from build123d import *

# Parameters (mm, degrees)
F1_DEPTH = 6.35
F2_R     = 3.175
F3_DEPTH = 6.35
F5_DEPTH = 5


with BuildPart() as f1:
    # F0 (on Front) → F1 (new body)
    with BuildSketch(Plane.XZ):
        with BuildLine():
            Line((69.85, 12.7), (0, 12.7))
            ThreePointArc((0, 12.7), (-12.7, 0), (0, -12.7))
            Line((0, -12.7), (69.85, -12.7))
            ThreePointArc((69.85, -12.7), (82.55, 0), (69.85, 12.7))
        make_face()
    extrude(amount=F1_DEPTH)

    # F2 (on face) → F3 (cut, through all)
    with BuildSketch(Plane.XZ.offset(6.35)):
        Circle(F2_R)
        with Locations((24, 0)):
            Circle(F2_R)
    extrude(amount=-F3_DEPTH, mode=Mode.SUBTRACT)

    # F4 (on face) → F5 (cut)
    with BuildSketch(Plane(origin=(0, 0, 0), x_dir=(-1, 0, 0), z_dir=(0, 1, 0))):
        with BuildLine():
            Line((-23.55792, 7.161368), (-69.23386, 9.981001))
            ThreePointArc((-69.23386, 9.981001), (-79.85, 0), (-69.23386, -9.981001))
            Line((-69.23386, -9.981001), (-23.55792, -7.161368))
            ThreePointArc((-23.55792, -7.161368), (-16.825, 0), (-23.55792, 7.161368))
        make_face()
    extrude(amount=-F5_DEPTH, mode=Mode.SUBTRACT)


solid = f1.part
Could you check a few things on this model? Use its own coordinates, in mm. A direction names the side the tool comes from. Give positions to 0.01 mm unless a question says otherwise; leave off trailing zeros. Order: outer loops, then holes, each group sorted by start corner. A loop starts at its lowest first (then second) coordinate and runs counter-clockwise, first axis right, second up. Notation, with made-up numbers: (79.5, 1.5) -> (86.5, 1.5) arc R19 ccw to (86.5, 22.5) -> close; hole circle Ø6 at (84, 57). An arc over 180 degrees is marked (long way). Return JSON: item names as keys, results as strings.
1. Imagine slicing it at C-C on x = 63. List the corners of the cut face in (y, z) for me, then the cut area to 3 significant figures.
Answer list:
{"outline": "(-6.35, -12.7) -> (0, -12.7) -> (0, -9.6) -> (-5, -9.6) -> (-5, 9.6) -> (0, 9.6) -> (0, 12.7) -> (-6.35, 12.7) -> close", "area": "65.3 mm2"}
2. I need wall thicknesses on line 1 (Z direction, x = 0, y = -1.5) (3 decimals); line 2 (X direction, y = -0.5, z = -2.5); line 3 (Y direction, x = 34.5, z = 4.5). Which ranges of each line are inside material? Lowest first, please. Write a range as from..to.
Answer list:
{"line 1": "z = -12.7..-3.175, 3.175..12.7", "line 2": "x = -12.45..-1.96, 1.96..17.27, 79.53..82.3", "line 3": "y = -6.35..-5"}
3. For pin 1 Ø10 at (x, z) = (64.5, -2) entering from +Y, with a flat end and sliding along its axis, tell me the tip position at first contact or that it passes through.
Answer list:
{"pin 1": "stops at y = -5"}
4. Imagine slicing it at B-B on z = 0. List the corners of the cut face in (x, y) for me (3 decimals), then the cut area to 3 significant figures.
Answer list:
{"outline": "(-12.7, -6.35) -> (-3.175, -6.35) -> (-3.175, 0) -> (-12.7, 0) -> close; (3.175, -6.35) -> (20.825, -6.35) -> (20.825, -5) -> (16.825, -5) -> (16.825, 0) -> (3.175, 0) -> close; (27.175, -6.35) -> (82.55, -6.35) -> (82.55, 0) -> (79.85, 0) -> (79.85, -5) -> (27.175, -5) -> close", "area": "241 mm2"}
5. Thinking about a two-plate mould opening in Z: for faces 1 (the cylindrical face through (82.547, -3.131, -0.279)), 2 (the flat face through (34, -6.35, 0)), 3 (the cylindrical face through (-0.69, -3.22, -3.1)), 4 (the flat face through (34, -3, -12.7)), which applies, pulls with the +Z half, pulls with the -Z half, needs draft (parallel to the pull), parting line crosses it, or undercut?
Answer list:
{"face 1": "parting line crosses it", "face 2": "needs draft", "face 3": "undercut", "face 4": "pulls with the -Z half"}
6. Imagine slicing it at A-A on y = -3.25. List the corners of the cut face in (x, z) for me (3 decimals), then the cut area to 3 significant figures.
Answer list:
{"outline": "(0, -12.7) -> (69.85, -12.7) arc R12.7 ccw to (69.85, 12.7) -> (0, 12.7) arc R12.7 ccw to start; hole circle Ø6.35 at (0, 0); hole (23.558, -7.161) -> (69.234, -9.981) arc R10 ccw (long way) to (69.234, 9.981) -> (23.558, 7.161) arc R7.175 ccw to start", "area": "1,220 mm2"}
7. Imagine slicing it at D-D on z = -4.5. List the corners of the cut face in (x, y) for me, then the cut area to 3 significant figures.
Answer list:
{"outline": "(-11.88, -6.35) -> (81.73, -6.35) -> (81.73, 0) -> (78.78, 0) -> (78.78, -5) -> (18.41, -5) -> (18.41, 0) -> (-11.88, 0) -> close", "area": "293 mm2"}
8. On a 3-axis mill with a long thin cutter (end or side, diameter ignored), from which of +Z, -Z, +X, -X, +Y, -Y can I reach the whole of each face in a straight line? I mean faces 5 (the flat face through (13, 0, 0)), 6 (the flat face through (46.08, -2.46, 8.55)). Say none if no direction works.
Answer list:
{"face 5": "+Z, -Z, +X, -X, +Y", "face 6": "+Y"}
